Solid Edge part; units mm, degrees
sketch "Sketch1" plane through (0, 0, 0) normal (0, 0, 1) x (1, 0, 0)
  circle A0 centre (0, 0) radius 7.8486
extrude "Protrusion1" add sketch "Sketch1" along normal blind 4.8006
sketch "Sketch2" plane through (0, 0, 0) normal (0, 0, -1) x (1, 0, 0)
  circle A0 centre (0, 0) radius 3.9688
extrude "Protrusion2" add sketch "Sketch2" along normal blind 14.2494
sketch "Sketch3" plane through (0, 0, -14.2494) normal (0, 0, -1) x (1, 0, 0)
  circle A0 centre (0, 0) radius 3.9685
extrude "Cutout1" cut sketch "Sketch3" against normal blind 14.2352 flip side to cut
chamfer "Chamfer_1" distance 0.5953 angle 45 1 edges at (-3.9685, 0, -14.2494)
sketch "Sketch4" plane through (0, 0, 4.8006) normal (0, 0, 1) x (1, 0, 0)
  line L0 (-1.3748, 2.3812) -> (1.3748, 2.3812)
  line L1 (2.7496, 0) -> (1.3748, 2.3812)
  line L2 (1.3748, -2.3812) -> (2.7496, 0)
  line L3 (-1.3748, -2.3812) -> (1.3748, -2.3812)
  line L4 (-2.7496, 0) -> (-1.3748, -2.3812)
  line L5 (-1.3748, 2.3812) -> (-2.7496, 0)
extrude "Cutout2" cut sketch "Sketch4" against normal blind 3.2004
sketch "Sketch5" plane through (0, 0, 0) normal (0, -1, 0) x (1, 0, 0)
  line L0 (7.8486, 4.8006) -> (3.6755, 0)
  line L1 (3.6755, 0) -> (7.8486, 0)
  line L2 (7.8486, 0) -> (7.8486, 4.8006)
revolve "RevolvedCutout1" cut sketch "Sketch5" angle 360 about axis through (0, 0, 14.0017) along (0, 0, -1)
properties part number "24101007"
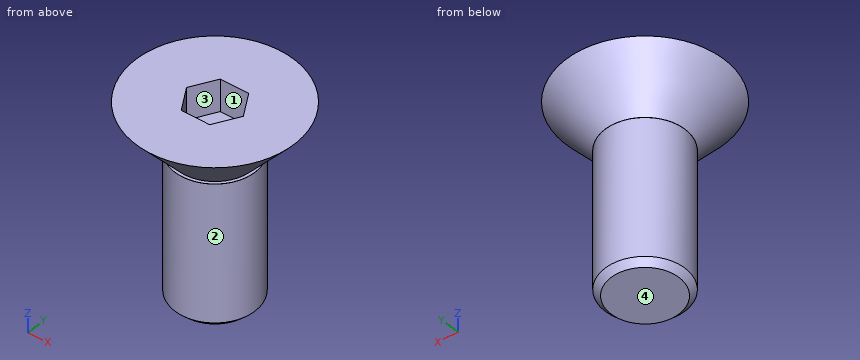
Geometry: final body of the model. Coordinates: model frame, mm. Face numbers are marked on the shaded views. Coordinates: 2 decimals unless noted, no trailing zeros. Order: outer loops, then holes, each group sorted by start corner. A loop starts at its lowest first (then second) coordinate and runs counter-clockwise, first axis right, second up.
(1) Section query C-C (z = -13). Return the cut outline in (x, y), plus the area to 3 significant figures.
(2) Material intervals for probe 1 along X at (y, z) = (-3, -8.75); probe 2 along Y at (x, z) = (0.25, -12.25); probe 3 along Z at (x, y) = (-3, -3.25), sorted ascending.
(3) First-contact query: pin 1 (4 mm diameter, centred on x = 1.5, y = 0.5, fed in from +Z); pin 2 (4 mm diameter, centred on x = -3, z = -2.5, fed in from +Y); pin 3 (4 mm diameter, centred on y = -0.5, z = 1, fed in from +X); pin 4 (0.8 mm diameter, centred on x = 0.5, z = 3.5, fed in from -Y). Flat tips, straight axial feed; report the tip coordinate or a pass-through.
(4) Section query A-A (z = 2). Return the cut outline in (x, y).
(5) Draft query along Y for the marked faces 1, 2, 3 and 4. Return one class per face: pulls with the +Y half, pulls with the -Y half, needs draft (parallel to the pull), parting line crosses it, or undercut.
Solution:
1. outline: circle Ø7.94 at (0, 0)
1. area: 49.5 mm2
2. probe 1: x = -2.6 to 2.6
2. probe 2: y = -3.96 to 3.96
2. probe 3: z = 0.86 to 4.8
3. pin 1: stops at z = 4.8
3. pin 2: stops at y = 3.84
3. pin 3: stops at x = 6.27
3. pin 4: stops at y = -7.05
4. outline: circle Ø10.83 at (0, 0); hole (-2.75, 0) - (-1.37, -2.38) - (1.37, -2.38) - (2.75, 0) - (1.37, 2.38) - (-1.37, 2.38) - close
5. face 1: undercut
5. face 2: parting line crosses it
5. face 3: undercut
5. face 4: needs draft
